from build123d import *

# Parameters (mm, degrees)
SKETCH1_W               = 100
SKETCH1_H               = 30
BOSS_EXTRUDE1_DEPTH     = 1.5
SKETCH2_W               = 80
SKETCH2_H               = 15
SKETCH2_W_2             = 77
SKETCH2_H_2             = 12
EXTRUDE_THIN1_DEPTH     = 0.1
SKETCH3_R               = 5
BOSS_EXTRUDE2_DEPTH     = 0.1
CUT_EXTRUDE1_DEPTH      = 53.226047141
CUT_EXTRUDE1_DEPTH_BACK = 53.226047141
SKETCH4_R               = 1.5
FILLET1_R               = 5


with BuildPart() as part:
    # Sketch1 → Boss-Extrude1 (new body)
    with BuildSketch(Plane.XY):
        Rectangle(SKETCH1_W, SKETCH1_H)
    extrude(amount=BOSS_EXTRUDE1_DEPTH)

    # Sketch2 → Extrude-Thin1 (add)
    with BuildSketch(Plane.XY.offset(1.5)):
        Rectangle(SKETCH2_W, SKETCH2_H)
        Rectangle(SKETCH2_W_2, SKETCH2_H_2, mode=Mode.SUBTRACT)
    extrude(amount=EXTRUDE_THIN1_DEPTH)

    # Sketch3 → Boss-Extrude2 (add)
    with BuildSketch(Plane.XY.offset(1.5)):
        with Locations((-35, 0)):
            Circle(SKETCH3_R)
        with Locations((35, 0)):
            Circle(SKETCH3_R)
    extrude(amount=BOSS_EXTRUDE2_DEPTH)

    # Sketch4 → Cut-Extrude1 (cut, two sides: drawn at the far end of the back side and taken through both)
    with BuildSketch(Plane.XY.offset(1.6).offset(-CUT_EXTRUDE1_DEPTH_BACK)):
        with Locations((-35, 0)):
            Circle(SKETCH4_R)
        with Locations((35, 0)):
            Circle(SKETCH4_R)
    extrude(amount=CUT_EXTRUDE1_DEPTH + CUT_EXTRUDE1_DEPTH_BACK, mode=Mode.SUBTRACT)

    # Fillet1
    # the kernel refuses this fillet: 5 mm, written as the material it adds along each edge
    with BuildSketch(Plane(origin=(38.5, -6, 1.5), x_dir=(0, 1, 0), z_dir=(0, 0, 1))) as fillet1_piece_1:
        with BuildLine():
            CenterArc((5, 4.288522873), FILLET1_R, 180, 59.059821395)
            Line((0, 4.288522873), (0, 0))
            Line((0, 0), (2.429285786, 0))
        make_face()
    extrude(amount=0.1)
    with BuildSketch(Plane(origin=(38.5, 6, 1.5), x_dir=(0, -1, 0), z_dir=(0, 0, 1))) as fillet1_piece_2:
        with BuildLine():
            CenterArc((5, -4.288522873), FILLET1_R, 120.940178605, 59.059821395)
            Line((0, -4.288522873), (0, 0))
            Line((0, 0), (2.429285786, 0))
        make_face()
    extrude(amount=0.1)
    with BuildSketch(Plane(origin=(-38.5, -6, 1.5), x_dir=(1, 0, 0), z_dir=(0, 0, 1))) as fillet1_piece_3:
        with BuildLine():
            CenterArc((4.288522873, 5), FILLET1_R, 210.940178605, 59.059821395)
            Line((0, 2.429285786), (0, 0))
            Line((0, 0), (4.288522873, 0))
        make_face()
    extrude(amount=0.1)
    with BuildSketch(Plane(origin=(-38.5, 6, 1.5), x_dir=(1, 0, 0), z_dir=(0, 0, 1))) as fillet1_piece_4:
        with BuildLine():
            CenterArc((4.288522873, -5), FILLET1_R, 90, 59.059821395)
            Line((0, -2.429285786), (0, 0))
            Line((0, 0), (4.288522873, 0))
        make_face()
    extrude(amount=0.1)
    # the kernel refuses this fillet: 5 mm, written as the material it takes off along each edge
    with BuildSketch(Plane(origin=(40, 7.5, 1.5), x_dir=(0, -1, 0), z_dir=(0, 0, 1)), Plane(origin=(40, -7.5, 1.5), x_dir=(-1, 0, 0), z_dir=(0, 0, 1)), Plane(origin=(-40, 7.5, 1.5), x_dir=(1, 0, 0), z_dir=(0, 0, 1))) as fillet1_2_piece_1:
        with BuildLine():
            CenterArc((FILLET1_R, -FILLET1_R), FILLET1_R, 90, 90)
            Line((0, -FILLET1_R), (0, 0))
            Line((0, 0), (FILLET1_R, 0))
        make_face()
    extrude(amount=12.6, mode=Mode.SUBTRACT)
    with BuildSketch(Plane(origin=(-40, -7.5, 1.5), x_dir=(1, 0, 0), z_dir=(0, 0, 1))) as fillet1_2_piece_2:
        with BuildLine():
            CenterArc((FILLET1_R, FILLET1_R), FILLET1_R, 180, 90)
            Line((0, FILLET1_R), (0, 0))
            Line((0, 0), (FILLET1_R, 0))
        make_face()
    extrude(amount=12.6, mode=Mode.SUBTRACT)
    with BuildSketch(Plane(origin=(-50, 15, -12.5), x_dir=(1, 0, 0), z_dir=(0, 0, 1)), Plane(origin=(-50, -15, -12.5), x_dir=(0, 1, 0), z_dir=(0, 0, 1))) as fillet1_2_piece_3:
        with BuildLine():
            CenterArc((FILLET1_R, -FILLET1_R), FILLET1_R, 90, 90)
            Line((0, -FILLET1_R), (0, 0))
            Line((0, 0), (FILLET1_R, 0))
        make_face()
    extrude(amount=26.5, mode=Mode.SUBTRACT)
    with BuildSketch(Plane(origin=(50, -15, -12.5), x_dir=(0, 1, 0), z_dir=(0, 0, 1)), Plane(origin=(50, 15, -12.5), x_dir=(-1, 0, 0), z_dir=(0, 0, 1))) as fillet1_2_piece_4:
        with BuildLine():
            CenterArc((FILLET1_R, FILLET1_R), FILLET1_R, 180, 90)
            Line((0, FILLET1_R), (0, 0))
            Line((0, 0), (FILLET1_R, 0))
        make_face()
    extrude(amount=26.5, mode=Mode.SUBTRACT)


solid = part.part
Read the model definition and answer for the solid it produces. Units are mm, in the model's axes. A direction names the side the tool comes from. Coordinates: 2 decimals unless noted, no trailing zeros. Write each loop counter-clockwise with the first axis right and the second up, starting at its lowest first coordinate (ties: lowest second). Pieces come first, ordered by that corner, then holes. Notation, with made-up numbers: M 68,-25.5 L 74,-25.5 A11 cw 74,-15.5 Z; hole C 75,-19.5 d2. An arc over 180 degrees is marked long. Use a Markdown table: item, result.
Q1. The part is cut by section B-B, the plane x = -13. Write down the section's boundary in (y, z), then the cut area to 3 significant figures.
Answer block:
| item | result |
|---|---|
| outline | M -15,0 L 15,0 L 15,1.5 L 7.5,1.5 L 7.5,1.6 L 6,1.6 L 6,1.5 L -6,1.5 L -6,1.6 L -7.5,1.6 L -7.5,1.5 L -15,1.5 Z |
| area | 45.3 mm2 |
Q2. The part is cut by section D-D, the plane y = 12. Write down the section's boundary in (x, z).
Answer block:
| item | result |
|---|---|
| outline | M -49.58,0 L 49.58,0 L 49.58,1.5 L -49.58,1.5 Z |
Q3. The part is cut by section C-C, the plane x = 41. Write down the section's boundary in (y, z).
Answer block:
| item | result |
|---|---|
| outline | M -15,0 L 15,0 L 15,1.5 L -15,1.5 Z |
Q4. Which of the six approach directions +Z, -Z, +X, -X, +Y, -Y give full straight-line access (tool end or side, diameter ignored) to faces 5 (the face through (-1, 0, 1.5)), 6 (the face through (-48, 14, 1))?
Answer block:
| item | result |
|---|---|
| face 5 | +Z |
| face 6 | +Z, -Z, -X, +Y |
Q5. The part is cut by section A-A, the plane y = 0. Write down the section's boundary in (x, z), then the cut area to 3 significant figures.
Answer block:
| item | result |
|---|---|
| outline | M -50,0 L -36.5,0 L -36.5,1.6 L -40,1.6 L -40,1.5 L -50,1.5 Z; M -33.5,0 L 33.5,0 L 33.5,1.6 L 30,1.6 L 30,1.5 L -30,1.5 L -30,1.6 L -33.5,1.6 Z; M 36.5,0 L 50,0 L 50,1.5 L 40,1.5 L 40,1.6 L 36.5,1.6 Z |
| area | 142 mm2 |
Q6. Straight lines are drawn through the part: L1, parallel to X at y = 0, z = 0.4; L2, parallel to Y at x = -35, z = 0.45; L3, parallel to Z at x = -20.5, y = 0.5. For each, find the intervals that lie inside material, in ascending order. Write a range as [from, to].
Answer block:
| item | result |
|---|---|
| L1 | x = [-50, -36.5], [-33.5, 33.5], [36.5, 50] |
| L2 | y = [-15, -1.5], [1.5, 15] |
| L3 | z = [0, 1.5] |
Q7. Determine the mould class of faces 1 (the face through (-36.2, -0.9, 0.8)), 2 (the face through (33.8, -0.9, 0.8)), 3 (the face through (-1, 0, 0)), 4 (the face through (48, -14, 1)) for opening direction X: released by +X, released by -X, zero draft, split by the parting line, or undercut.
Answer block:
| item | result |
|---|---|
| face 1 | undercut |
| face 2 | undercut |
| face 3 | zero draft |
| face 4 | released by +X |
